Verification items for the finished model (mm, model axes). A direction names the side the tool comes from. Coordinates: 2 decimals unless noted, no trailing zeros. Order: outer loops, then holes, each group sorted by start corner. A loop starts at its lowest first (then second) coordinate and runs counter-clockwise, first axis right, second up. Notation, with made-up numbers: M -2,41 L 46,41 A15 ccw 46,63 Z; hole C 72.25,64 d5. An arc over 180 degrees is marked long. Write item = value, one per line.
```python
from build123d import *

# Parameters (mm, degrees)
SKETCH_1_W      = 15.25
SKETCH_1_H      = 141.25
SKETCH_1_R      = 1.6
EXTRUDE_1_DEPTH = 5
SKETCH_2_W      = 21.25
SKETCH_2_H      = 147.25
SKETCH_2_W_2    = 15.25
SKETCH_2_H_2    = 141.25
EXTRUDE_2_DEPTH = 10
CHAMFER_1_SIZE  = 2


with BuildPart() as part:
    # ｽｹｯﾁ1 → ﾎﾞｽ - 押し出し1 (new body)
    with BuildSketch(Plane(origin=(0, 5, 0), x_dir=(1, 0, 0), z_dir=(0, 1, 0))):
        Rectangle(SKETCH_1_W, SKETCH_1_H)
        with Locations(Location((0, -30, 0), (0, 0, 180))):
            Circle(SKETCH_1_R, mode=Mode.SUBTRACT)
        with Locations(Location((0, 65.5, 0), (0, 0, 180))):
            Circle(SKETCH_1_R, mode=Mode.SUBTRACT)
        with Locations(Location((0, 45.5, 0), (0, 0, 180))):
            Circle(SKETCH_1_R, mode=Mode.SUBTRACT)
        with Locations(Location((0, -45.5, 0), (0, 0, 180))):
            Circle(SKETCH_1_R, mode=Mode.SUBTRACT)
        with Locations(Location((0, 30, 0), (0, 0, 180))):
            Circle(SKETCH_1_R, mode=Mode.SUBTRACT)
        with Locations(Location((0, -65.5, 0), (0, 0, 180))):
            Circle(SKETCH_1_R, mode=Mode.SUBTRACT)
    extrude(amount=EXTRUDE_1_DEPTH)

    # ｽｹｯﾁ2 → ﾎﾞｽ - 押し出し2 (add)
    with BuildSketch(Plane(origin=(0, 10, 0), x_dir=(1, 0, 0), z_dir=(0, 1, 0))):
        Rectangle(SKETCH_2_W, SKETCH_2_H)
        Rectangle(SKETCH_2_W_2, SKETCH_2_H_2, mode=Mode.SUBTRACT)
    extrude(amount=-EXTRUDE_2_DEPTH)

    # 面取り1
    chamfer_1_edges = [part.edges().sort_by_distance(p)[0] for p in [
        (-7.625, 0, 0),
        (0, 0, 70.625),
        (7.625, 0, 0),
        (0, 0, -70.625),
    ]]
    chamfer(chamfer_1_edges, length=CHAMFER_1_SIZE)


solid = part.part
```
Item 1: Sectioned sample at A-A, the plane x = 0. Give the number of separate pieces and of enclosed holes in the cut face, then the cut area to 3 significant figures.
Report:
separate_pieces = 7
enclosed_holes = 0
area = 666 mm^2
Item 2: Sectioned sample at D-D, the plane z = -25.5. Enter the section's corners in (x, y) (3 decimals).
Report:
outline = M -10.625,0 L -9.625,0 L -7.625,2 L -7.625,5 L 7.625,5 L 7.625,2 L 9.625,0 L 10.625,0 L 10.625,10 L -10.625,10 Z
Item 3: Sectioned sample at C-C, the plane z = -45.5. Enter the section's corners in (x, y) (3 decimals), then the cut area to 3 significant figures.
Report:
outline = M -10.625,0 L -9.625,0 L -7.625,2 L -7.625,5 L -1.6,5 L -1.6,10 L -10.625,10 Z; M 1.6,5 L 7.625,5 L 7.625,2 L 9.625,0 L 10.625,0 L 10.625,10 L 1.6,10 Z
area = 116 mm^2
Item 4: Scan lines: L1, parallel to X at y = 6.9, z = 65.5 (3 decimals); L2, parallel to Z at x = 5.5, y = 2 (3 decimals); L3, parallel to Y at x = -7, z = -47.5. Record each from-to range of solid material in increasing order. Write a range as from..to.
Report:
L1 = -10.625..-1.6, 1.6..10.625
L2 = -73.625..-70.625, 70.625..73.625
L3 = 5..10
Item 5: Gauge pin test, flat end, axial feed: pin 1 (4 mm diameter, centred on x = 0, z = 30, fed in from -Y). Record the tip position at first contact, or that the pin passes through.
Report:
pin_1 = 5
Item 6: Tool access check on faces 1 (the flat face through (0, 4, -70.625)), 2 (the cylindrical face through (0.208, 7.465, 31.586)). Record the directions out of +Z, -Z, +X, -X, +Y, -Y that give a thin tool (end or side, any length) a straight path to the whole face; none if there is none.
Report:
face_1 = -Y
face_2 = +Y, -Y
Item 7: Sectioned sample at B-B, the plane y = 8. Enter the section's corners in (x, z) (3 decimals).
Report:
outline = M -10.625,-73.625 L 10.625,-73.625 L 10.625,73.625 L -10.625,73.625 Z; hole C 0,-65.5 d3.2; hole C 0,-45.5 d3.2; hole C 0,-30 d3.2; hole C 0,30 d3.2; hole C 0,45.5 d3.2; hole C 0,65.5 d3.2
Item 8: Release check for a two-part mould opening along Z. For faces 3 (the flat face through (0, 5, 73.625)), 4 (the flat face through (-10.625, 5, 1)), 5 (the cylindrical face through (0.208, 7.465, -63.914)) record: pulls with the +Z half, pulls with the -Z half, needs draft (parallel to the pull), parting line crosses it, or undercut.
Report:
face_3 = pulls with the +Z half
face_4 = needs draft
face_5 = undercut
